The model under review builds one solid part; all positions refer to its coordinate system, in mm. Face numbers are marked on the shaded views. Round coordinates to 2 decimals unless told otherwise and drop trailing zeros. Write each loop counter-clockwise with the first axis right and the second up, starting at its lowest first coordinate (ties: lowest second). Pieces come first, ordered by that corner, then holes. Notation, with made-up numbers: (-9.75, 28) -> (0.25, 28) arc R10 ccw to (0.25, 38) -> close; hole circle Ø1 at (42, 61.25). An arc over 180 degrees is marked (long way). Use CSV: the item, a comma, the result in double quotes. Start each with the question number.
1) Take a section at C-C, the plane y = 6.25. Give the boundary of the cut face in (x, z) (3 decimals).
2) Wall thickness on probe 1 along X at (y, z) = (1.5, 0) (3 decimals); probe 2 along Z at (x, y) = (4.25, 3): over which ranges is each line inside the solid? List them lowest first. Write a range as [from, to].
3) For pin 1 Ø3 at (y, z) = (-2.5, -6) entering from +X (3 decimals), flat-tipped, find the tip position at first contact; note if it passes through.
4) Mouldability with a two-part tool opening along X and no side actions: class the marked faces 1, 2 and 3 as released by +X, released by -X, zero draft, split by the parting line, or undercut.
5) Take a section at B-B, the plane z = 0. Give the boundary of the cut face in (x, y) (1 decimal), then the cut area to 3 significant figures.
6) Take a section at A-A, the plane x = 0. Give the boundary of the cut face in (y, z) (1 decimal).
from build123d import *

# Parameters (mm, degrees)
ESQUISSE2_R        = 9.525
ESQUISSE2_R_2      = 4.8514
BOSS_EXTRU_1_DEPTH = 7.9375
CONG_2_R           = 0.5


with BuildPart() as part:
    # Esquisse2 → Boss.-Extru.1 (new body, symmetric)
    with BuildSketch(Plane(origin=(0, 0, 0), x_dir=(1, 0, 0), z_dir=(0, 1, 0))):
        Circle(ESQUISSE2_R)
        Circle(ESQUISSE2_R_2, mode=Mode.SUBTRACT)
    extrude(amount=BOSS_EXTRU_1_DEPTH, both=True)

    # Congé2
    cong_2_edges = [part.edges().sort_by_distance(p)[0] for p in [
        (-9.525, -7.9375, 0),
        (-9.525, 7.9375, 0),
        (-4.8514, -7.9375, 0),
        (-4.8514, 7.9375, 0),
    ]]
    fillet(cong_2_edges, radius=CONG_2_R)


solid = part.part
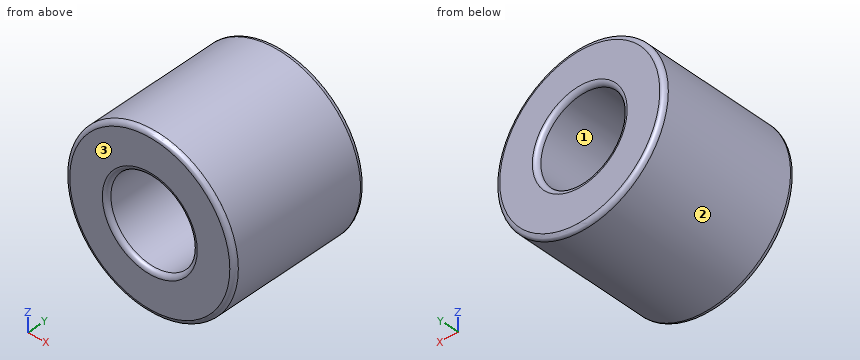
Values found:
1,outline,"circle Ø19.05 at (0, 0); hole circle Ø9.703 at (0, 0)"
2,probe 1,"[-9.525, -4.851], [4.851, 9.525]"
2,probe 2,"[-8.52, -2.34], [2.34, 8.52]"
3,pin 1,"x = 8.395"
4,face 1,"undercut"
4,face 2,"split by the parting line"
4,face 3,"zero draft"
5,outline,"(-9.5, -7.4) arc R0.5 ccw to (-9, -7.9) -> (-5.4, -7.9) arc R0.5 ccw to (-4.9, -7.4) -> (-4.9, 7.4) arc R0.5 ccw to (-5.4, 7.9) -> (-9, 7.9) arc R0.5 ccw to (-9.5, 7.4) -> close; (4.9, -7.4) arc R0.5 ccw to (5.4, -7.9) -> (9, -7.9) arc R0.5 ccw to (9.5, -7.4) -> (9.5, 7.4) arc R0.5 ccw to (9, 7.9) -> (5.4, 7.9) arc R0.5 ccw to (4.9, 7.4) -> close"
5,area,"148 mm²"
6,outline,"(-7.9, -9) arc R0.5 ccw to (-7.4, -9.5) -> (7.4, -9.5) arc R0.5 ccw to (7.9, -9) -> (7.9, -5.4) arc R0.5 ccw to (7.4, -4.9) -> (-7.4, -4.9) arc R0.5 ccw to (-7.9, -5.4) -> close; (-7.9, 5.4) arc R0.5 ccw to (-7.4, 4.9) -> (7.4, 4.9) arc R0.5 ccw to (7.9, 5.4) -> (7.9, 9) arc R0.5 ccw to (7.4, 9.5) -> (-7.4, 9.5) arc R0.5 ccw to (-7.9, 9) -> close"
